Source: CAD feature listing. Evaluate the final solid. Frame: model axes, mm. Face numbers are marked on the shaded views. Give positions to 0.01 mm unless a question says otherwise; leave off trailing zeros. Write each loop counter-clockwise with the first axis right and the second up, starting at its lowest first coordinate (ties: lowest second). Pieces come first, ordered by that corner, then holes. Notation, with made-up numbers: (46.5, 49) -> (83.5, 49) arc R12 cw to (83.5, 57) -> close; hole circle Ø1 at (30, 78). An arc over 180 degrees is marked (long way). Use one line per item in the form item = value. Start each with the question number.
(1) Draft query along X for the marked faces 1 and 2. Return one class per face: pulls with the +X half, pulls with the -X half, needs draft (parallel to the pull), parting line crosses it, or undercut.
(2) First-contact query: P1, Ø6.5, axis at x = 9.5, y = -10, coming from the +Z side; P2, Ø10, axis at x = -48, y = -9.5, coming from the +Z side; P3, Ø1.5, axis at x = -6.5, z = 2.5, coming from the -Y side. Flat tips, straight axial feed; report the tip coordinate or a pass-through.
(3) Cut plane B-B, the plane x = -10.5. Output: boundary loops of the cut face in (y, z), and give its area (3 significant figures).
(4) Cut plane A-A, the plane y = -8.5. Output: boundary loops of the cut face in (x, z).
(5) Cut plane C-C, the plane x = -60. Output: boundary loops of the cut face in (y, z).
(6) Material intervals for line 1 along X through (y, z) = (-14, 1.1); line 2 along Y through (x, z) = (-12, 3.75); line 3 along Z through (x, y) = (18, -11.25), sorted ascending. Write a range as from..to.
from build123d import *

# Parameters (mm, degrees)
SKETCH007_W     = 56
SKETCH007_H     = 23
PAD004_DEPTH    = 4
SKETCH008_W     = 53
SKETCH008_H     = 25.379599
POCKET003_DEPTH = 3
SKETCH009_R     = 1.5
PAD005_DEPTH    = 70


with BuildPart() as part:
    # Sketch007 → Pad004 (new body)
    with BuildSketch(Plane.XY):
        Rectangle(SKETCH007_W, SKETCH007_H)
    extrude(amount=PAD004_DEPTH)

    # Sketch008 (on Face6 of Pad004) → Pocket003 (cut)
    with BuildSketch(Plane.XY.offset(4)):
        with Locations((0, -2.689799)):
            Rectangle(SKETCH008_W, SKETCH008_H)
    extrude(amount=-POCKET003_DEPTH, mode=Mode.SUBTRACT)

    # Sketch009 (on Face2 of Pocket003) → Pad005 (join)
    with BuildSketch(Plane(origin=(-28, 0, 0), x_dir=(0, -1, 0), z_dir=(-1, 0, 0))):
        with Locations((5.5, 1.5)):
            Circle(SKETCH009_R)
    extrude(amount=PAD005_DEPTH)


with BuildPart() as part_1:
    # Body002 placement: moved
    add(part.part.moved(Location((0, -6.75, 0))))


solid = part_1.part
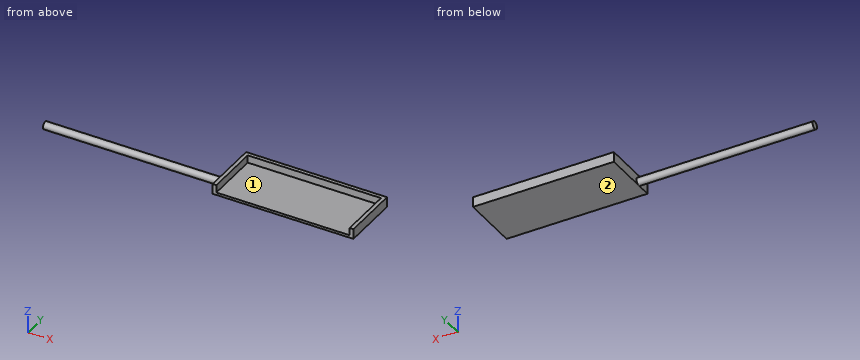
Geometry says:
q1.face_1 = undercut
q1.face_2 = needs draft
q2.P1 = 1
q2.P2 = 3
q2.P3 = 3.25
q3.outline = (-18.25, 0) -> (4.75, 0) -> (4.75, 4) -> (3.25, 4) -> (3.25, 1) -> (-18.25, 1) -> close
q3.area = 27.5 mm^2
q4.outline = (-28, 0) -> (28, 0) -> (28, 4) -> (26.5, 4) -> (26.5, 1) -> (-26.5, 1) -> (-26.5, 4) -> (-28, 4) -> close
q5.outline = circle Ø3 at (-12.25, 1.5)
q6.line_1 = -28..-26.5, 26.5..28
q6.line_2 = 3.25..4.75
q6.line_3 = 0..1
